Geometry check sheet. Reference: the model listing, model coordinates, mm. Round coordinates to 2 decimals unless told otherwise and drop trailing zeros. Loops run counter-clockwise (first coordinate to the right, second up) from the corner with the lowest first, then second, coordinate; pieces in that order, holes last. Notation, with made-up numbers: (-29, 31) -> (21, 31) arc R16 cw to (21, 38) -> close; hole circle Ø11 at (68, 26.5). An arc over 180 degrees is marked (long way). Use a Markdown table: item, result. Add a question column.
Q1. Sectioned sample at A-A, the plane x = 166. Enter the section's corners in (y, z).
Q2. Sectioned sample at B-B, the plane y = -3.75. Enter the section's corners in (x, z), then the cut area to 3 significant figures.
Q3. Material ranges on L1, parallel to Z at x = 222, y = 3.5; L2, parallel to Z at x = 53.5, y = 1; L3, parallel to Y at x = 52, z = 5.25, recorded low to high.
Autodesk Inventor part; units mm, degrees
ref_plane "YZ Plane" through (0, 0, 0) normal (1, 0, 0) x (0, 1, 0)
ref_plane "XZ Plane" through (0, 0, 0) normal (0, 1, 0) x (-1, 0, 0)
ref_plane "XY Plane" through (0, 0, 0) normal (0, 0, 1) x (1, 0, 0)
sketch "Sketch1" plane through (0, 0, 0) normal (1, 0, 0) x (0, 1, 0)
  line L0 (6.35, 3.6662) -> (6.35, -3.6662)
  line L1 (6.35, -3.6662) -> (0, -7.3323)
  line L2 (0, -7.3323) -> (-6.35, -3.6662)
  line L3 (-6.35, -3.6662) -> (-6.35, 3.6662)
  line L4 (-6.35, 3.6662) -> (0, 7.3323)
  line L5 (0, 7.3323) -> (6.35, 3.6662)
  point P0 (0, 0)
  dimension "d0" = 12.7
  dimension "d1" = 12.7
  dimension "d2" = 12.7
  dimension "d3" = 6.35
  dimension "d4" = 120
  dimension "d5" = 120
  dimension "d6" = 6.35
  dimension "d7" = 6.35
extrude "Extrusion1" add sketch "Sketch1" along normal blind 450.85
properties part number "0.5 hex shaft"
Values:
| question | item | result |
|---|---|---|
| 1 | outline | (-6.35, -3.67) -> (0, -7.33) -> (6.35, -3.67) -> (6.35, 3.67) -> (0, 7.33) -> (-6.35, 3.67) -> close |
| 2 | outline | (0, -5.17) -> (450.85, -5.17) -> (450.85, 5.17) -> (0, 5.17) -> close |
| 2 | area | 4,660 mm^2 |
| 3 | L1 | -5.31 to 5.31 |
| 3 | L2 | -6.75 to 6.75 |
| 3 | L3 | -3.61 to 3.61 |
